For this review, use the dimensioned drawing (mm, ordinates from the lowest corner) and the shaded views. A direction names the side the tool comes from. Give positions to 0.01 mm unless a question says otherwise; leave off trailing zeros. Order: outer loops, then holes, each group sorted by start corner. A loop starts at its lowest first (then second) coordinate and runs counter-clockwise, first axis right, second up. Notation, with made-up numbers: (-1.5, -25) - (45.5, -25) arc R24 cw to (45.5, -9) - close; hole circle Ø4 at (3.25, 24). An arc over 180 degrees is marked (long way). Answer as CSV lines item,"result". Start each with the question number.
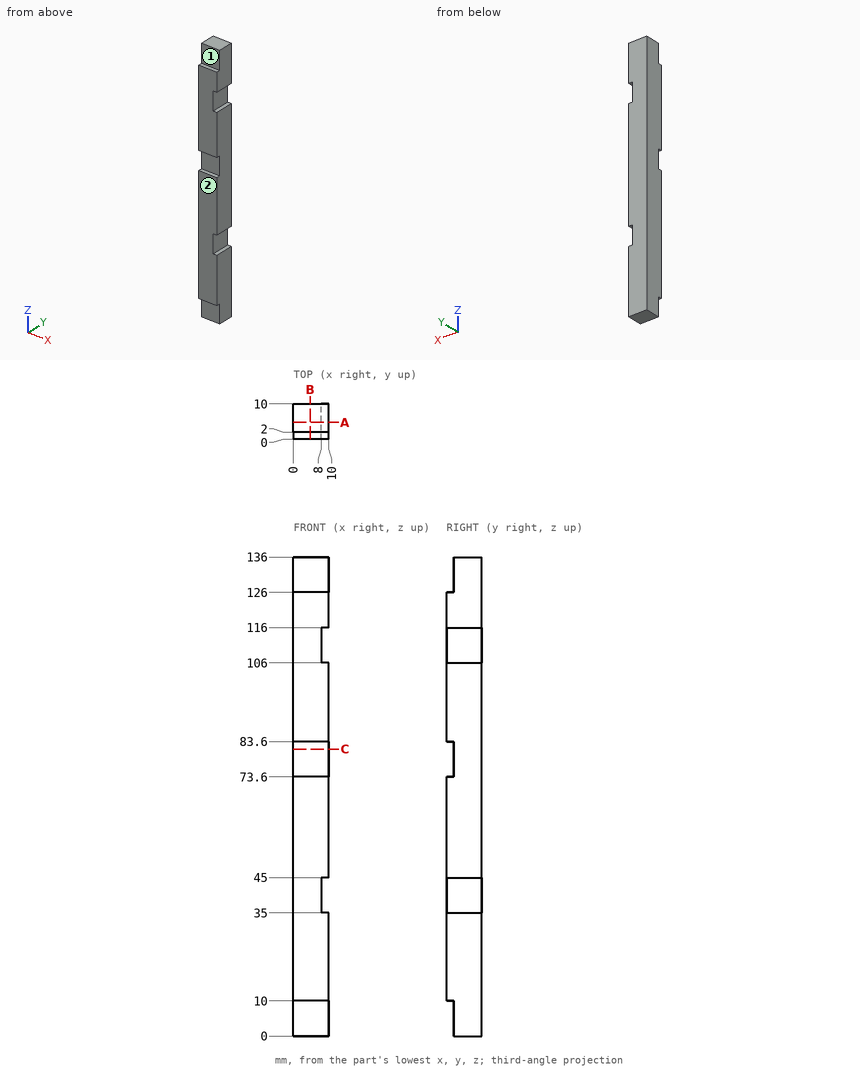
Item 1: Take a section at A-A on y = 4.75. Write out the cut boundary in (x, z).
Item 2: Take a section at C-C on z = 81.5. Write out the cut boundary in (x, y).
Item 3: Clearance check with flat-ended pins moving along their axes: pin 1 (0.6 mm diameter, centred on x = 4.5, y = 1, fed in from -Z); pin 2 (1 mm diameter, centred on x = 5, y = 1, fed in from +Z); pin 3 (3 mm diameter, centred on y = 6.5, z = 111, fed in from +X). State where each tip first meets the part, or that it passes through.
Item 4: For line 1 along Z through (x, y) = (9.5, 4.5); line 2 along Y through (x, z) = (8, 81.5); line 3 along Z through (x, y) = (7.5, 1), list the stretches that pass through material, from the lowest coordinate up.
Item 5: Take a section at B-B on x = 4.75. Write out the cut boundary in (y, z).
Item 6: Machinability: for the marked faces 1 and 2, which of the approach directions +Z, -Z, +X, -X, +Y, -Y give a long, thin tool a straight path to every point of the face, cutting with its end or side? Answer none if there is none.
Data:
1,outline,"(0, 0) - (10, 0) - (10, 35) - (8, 35) - (8, 45) - (10, 45) - (10, 106) - (8, 106) - (8, 116) - (10, 116) - (10, 136) - (0, 136) - close"
2,outline,"(0, 2) - (10, 2) - (10, 10) - (0, 10) - close"
3,pin 1,"stops at z = 10"
3,pin 2,"stops at z = 126"
3,pin 3,"stops at x = 8"
4,line 1,"z = 0 to 35, 45 to 106, 116 to 136"
4,line 2,"y = 2 to 10"
4,line 3,"z = 10 to 73.6, 83.6 to 126"
5,outline,"(0, 10) - (2, 10) - (2, 0) - (10, 0) - (10, 136) - (2, 136) - (2, 126) - (0, 126) - (0, 83.6) - (2, 83.6) - (2, 73.6) - (0, 73.6) - close"
6,face 1,"+Z, +X, -X, -Y"
6,face 2,"+Z, -Z, +X, -X, -Y"
